Could you check a few things on this model? Use its own coordinates, in mm. Round coordinates to 2 decimals unless told otherwise and drop trailing zeros. Answer in a Markdown table with one row per item.
from build123d import *

# Parameters (mm, degrees)
SKETCH_1_R      = 2.103037388
EXTRUDE_1_DEPTH = 600


with BuildPart() as part:
    # 草图1 → 凸台-拉伸1 (new body)
    with BuildSketch(Plane.XY):
        with BuildLine():
            Line((-32.248557314, -0.229845073), (-32.248557314, -1.030984477))
            Line((-32.248557314, -1.030984477), (-33.250003689, -1.030984477))
            Line((-33.250003689, -1.030984477), (-33.250003689, -6.238394755))
            ThreePointArc((-33.250003689, -6.238394755), (-32.949991565, -6.938952391), (-32.24382973, -7.225524788))
            Line((-32.24382973, -7.225524788), (-27.078556151, -7.225524788))
            Line((-27.078556151, -7.225524788), (-27.078556151, -6.224078413))
            Line((-27.078556151, -6.224078413), (-26.277399051, -6.224078413))
            Line((-26.277399051, -6.224078413), (-26.277399051, -5.212715786))
            Line((-26.277399051, -5.212715786), (-29.27300496, -5.212715786))
            Line((-29.27300496, -5.212715786), (-29.27300496, -4.211495229))
            Line((-29.27300496, -4.211495229), (-26.279632969, -1.225390538))
            Line((-26.279632969, -1.225390538), (-20.24902045, -1.225390538))
            Line((-20.24902045, -1.225390538), (-17.255648459, -4.211495229))
            Line((-17.255648459, -4.211495229), (-17.255648459, -5.212715786))
            Line((-17.255648459, -5.212715786), (-20.251254368, -5.212715786))
            Line((-20.251254368, -5.212715786), (-20.251254368, -6.224078413))
            Line((-20.251254368, -6.224078413), (-19.450097268, -6.224078413))
            Line((-19.450097268, -6.224078413), (-19.450097268, -7.225524788))
            Line((-19.450097268, -7.225524788), (-7.064233131, -7.225524788))
            Line((-7.064233131, -7.225524788), (-7.064233131, -6.224078413))
            Line((-7.064233131, -6.224078413), (-6.263076031, -6.224078413))
            Line((-6.263076031, -6.224078413), (-6.263076031, -5.212715786))
            Line((-6.263076031, -5.212715786), (-9.25868194, -5.212715786))
            Line((-9.25868194, -5.212715786), (-9.25868194, -4.211495229))
            Line((-9.25868194, -4.211495229), (-6.265309949, -1.225390538))
            Line((-6.265309949, -1.225390538), (-0.234697429, -1.225390538))
            Line((-0.234697429, -1.225390538), (2.758674561, -4.211495229))
            Line((2.758674561, -4.211495229), (2.758674561, -5.212715786))
            Line((2.758674561, -5.212715786), (-0.236931348, -5.212715786))
            Line((-0.236931348, -5.212715786), (-0.236931348, -6.224078413))
            Line((-0.236931348, -6.224078413), (0.564225752, -6.224078413))
            Line((0.564225752, -6.224078413), (0.564225752, -7.225524788))
            Line((0.564225752, -7.225524788), (12.945482254, -7.225524788))
            Line((12.945482254, -7.225524788), (12.945482254, -6.219120287))
            Line((12.945482254, -6.219120287), (13.751246989, -6.219120287))
            Line((13.751246989, -6.219120287), (13.751246989, -5.212715786))
            Line((13.751246989, -5.212715786), (10.755641081, -5.212715786))
            Line((10.755641081, -5.212715786), (10.755641081, -4.211495229))
            Line((10.755641081, -4.211495229), (13.749013071, -1.225390538))
            Line((13.749013071, -1.225390538), (19.779625591, -1.225390538))
            Line((19.779625591, -1.225390538), (22.772997581, -4.211495229))
            Line((22.772997581, -4.211495229), (22.772997581, -5.212715786))
            Line((22.772997581, -5.212715786), (19.772784037, -5.212715786))
            Line((19.772784037, -5.212715786), (19.772784037, -6.219120287))
            Line((19.772784037, -6.219120287), (20.573941137, -6.219120287))
            Line((20.573941137, -6.219120287), (20.573941137, -7.225524788))
            Line((20.573941137, -7.225524788), (25.743822351, -7.225524788))
            ThreePointArc((25.743822351, -7.225524788), (26.449984187, -6.938952391), (26.749996311, -6.238394755))
            Line((26.749996311, -6.238394755), (26.749996311, -1.030984477))
            Line((26.749996311, -1.030984477), (25.748549936, -1.030984477))
            Line((25.748549936, -1.030984477), (25.748549936, -0.229827377))
            Line((25.748549936, -0.229827377), (24.761302481, -0.229827377))
            Line((24.761302481, -0.229827377), (24.761302481, -3.234203038))
            Line((24.761302481, -3.234203038), (23.759856106, -3.234203038))
            Line((23.759856106, -3.234203038), (20.770104831, -0.237175589))
            Line((20.770104831, -0.237175589), (20.770104831, 5.786126014))
            Line((20.770104831, 5.786126014), (23.759856106, 8.783153462))
            Line((23.759856106, 8.783153462), (24.761302481, 8.783153462))
            Line((24.761302481, 8.783153462), (24.761302481, 5.778777801))
            Line((24.761302481, 5.778777801), (25.748549936, 5.778777801))
            Line((25.748549936, 5.778777801), (25.748549936, 6.579934901))
            Line((25.748549936, 6.579934901), (26.749996311, 6.579934901))
            Line((26.749996311, 6.579934901), (26.749996311, 11.768212512))
            ThreePointArc((26.749996311, 11.768212512), (26.456722319, 12.481138347), (25.743822351, 12.774475212))
            Line((25.743822351, 12.774475212), (20.573941137, 12.774475212))
            Line((20.573941137, 12.774475212), (20.573941137, 11.768070711))
            Line((20.573941137, 11.768070711), (19.772784037, 11.768070711))
            Line((19.772784037, 11.768070711), (19.772784037, 10.761666211))
            Line((19.772784037, 10.761666211), (22.772997581, 10.761666211))
            Line((22.772997581, 10.761666211), (22.772997581, 9.760445653))
            Line((22.772997581, 9.760445653), (19.779625591, 6.774340962))
            Line((19.779625591, 6.774340962), (13.749013071, 6.774340962))
            Line((13.749013071, 6.774340962), (10.755641081, 9.760445653))
            Line((10.755641081, 9.760445653), (10.755641081, 10.761666211))
            Line((10.755641081, 10.761666211), (13.746639354, 10.761666211))
            Line((13.746639354, 10.761666211), (13.746639354, 11.768070711))
            Line((13.746639354, 11.768070711), (12.945482254, 11.768070711))
            Line((12.945482254, 11.768070711), (12.945482254, 12.774475212))
            Line((12.945482254, 12.774475212), (0.564225752, 12.774475212))
            Line((0.564225752, 12.774475212), (0.564225752, 11.773028837))
            Line((0.564225752, 11.773028837), (-0.236931348, 11.773028837))
            Line((-0.236931348, 11.773028837), (-0.236931348, 10.761666211))
            Line((-0.236931348, 10.761666211), (2.758674561, 10.761666211))
            Line((2.758674561, 10.761666211), (2.758674561, 9.760445653))
            Line((2.758674561, 9.760445653), (-0.234697429, 6.774340962))
            Line((-0.234697429, 6.774340962), (-6.265309949, 6.774340962))
            Line((-6.265309949, 6.774340962), (-9.25868194, 9.760445653))
            Line((-9.25868194, 9.760445653), (-9.25868194, 10.761666211))
            Line((-9.25868194, 10.761666211), (-6.263076031, 10.761666211))
            Line((-6.263076031, 10.761666211), (-6.263076031, 11.773028837))
            Line((-6.263076031, 11.773028837), (-7.064233131, 11.773028837))
            Line((-7.064233131, 11.773028837), (-7.064233131, 12.774475212))
            Line((-7.064233131, 12.774475212), (-19.450097268, 12.774475212))
            Line((-19.450097268, 12.774475212), (-19.450097268, 11.773028837))
            Line((-19.450097268, 11.773028837), (-20.251254368, 11.773028837))
            Line((-20.251254368, 11.773028837), (-20.251254368, 10.761666211))
            Line((-20.251254368, 10.761666211), (-17.255648459, 10.761666211))
            Line((-17.255648459, 10.761666211), (-17.255648459, 9.760445653))
            Line((-17.255648459, 9.760445653), (-20.24902045, 6.774340962))
            Line((-20.24902045, 6.774340962), (-26.279632969, 6.774340962))
            Line((-26.279632969, 6.774340962), (-29.27300496, 9.760445653))
            Line((-29.27300496, 9.760445653), (-29.27300496, 10.761666211))
            Line((-29.27300496, 10.761666211), (-26.277399051, 10.761666211))
            Line((-26.277399051, 10.761666211), (-26.277399051, 11.773028837))
            Line((-26.277399051, 11.773028837), (-27.078556151, 11.773028837))
            Line((-27.078556151, 11.773028837), (-27.078556151, 12.774475212))
            Line((-27.078556151, 12.774475212), (-32.24382973, 12.774475212))
            ThreePointArc((-32.24382973, 12.774475212), (-32.956729698, 12.481138347), (-33.250003689, 11.768212512))
            Line((-33.250003689, 11.768212512), (-33.250003689, 6.560802234))
            Line((-33.250003689, 6.560802234), (-32.248557314, 6.560802234))
            Line((-32.248557314, 6.560802234), (-32.248557314, 5.759645134))
            Line((-32.248557314, 5.759645134), (-31.261309859, 5.759645134))
            Line((-31.261309859, 5.759645134), (-31.261309859, 8.764020795))
            Line((-31.261309859, 8.764020795), (-30.259863484, 8.764020795))
            Line((-30.259863484, 8.764020795), (-27.27011221, 5.766993347))
            Line((-27.27011221, 5.766993347), (-27.27011221, -0.237175589))
            Line((-27.27011221, -0.237175589), (-30.259863484, -3.234203038))
            Line((-30.259863484, -3.234203038), (-31.261309859, -3.234203038))
            Line((-31.261309859, -3.234203038), (-31.261309859, -0.229845073))
            Line((-31.261309859, -0.229845073), (-32.248557314, -0.229845073))
        make_face()
        with Locations((-3.250003689, 2.774475212)):
            Circle(SKETCH_1_R, mode=Mode.SUBTRACT)
        with Locations((-23.250003689, 2.774475212)):
            Circle(SKETCH_1_R, mode=Mode.SUBTRACT)
        with Locations((16.749996311, 2.774475212)):
            Circle(SKETCH_1_R, mode=Mode.SUBTRACT)
        Polygon((-19.258541209, 5.786126014), (-19.258541209, -0.237175589), (-15.26734356, -4.238086639), (-15.26734356, -5.22228212), (-11.246986839, -5.22228212), (-11.246986839, -4.238086639), (-7.25578919, -0.237175589), (-7.25578919, 2.774475212), (-7.25578919, 5.786126014), (-11.246986839, 9.787037063), (-11.246986839, 10.771232544), (-15.26734356, 10.771232544), (-15.26734356, 9.787037063), align=None, mode=Mode.SUBTRACT)
        Polygon((4.74697946, -5.22228212), (8.767336181, -5.22228212), (8.767336181, -4.238086639), (12.758533831, -0.237175589), (12.758533831, 2.774475212), (12.758533831, 5.786126014), (8.767336181, 9.787037063), (8.767336181, 10.771232544), (4.74697946, 10.771232544), (4.74697946, 9.787037063), (0.755781811, 5.786126014), (0.755781811, 2.774475212), (0.755781811, -0.237175589), (4.74697946, -4.238086639), align=None, mode=Mode.SUBTRACT)
    extrude(amount=EXTRUDE_1_DEPTH)


solid = part.part
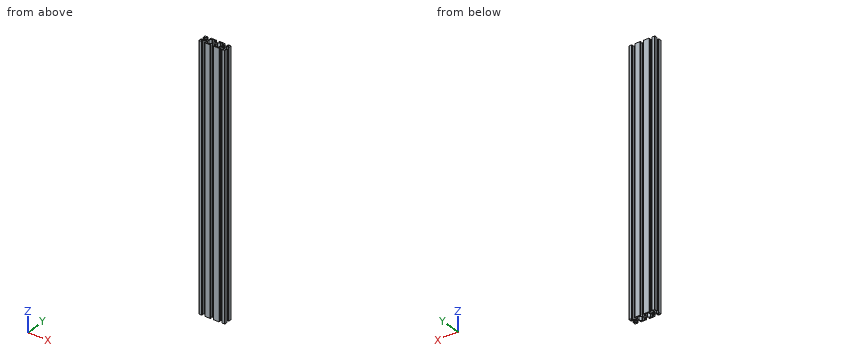
1) Imagine slicing it at A-A, the plane z = 432. Count the separate pieces of the cut face and the enclosed holes in it, plus the area to 3 significant figures.
Findings:
| item | result |
|---|---|
| separate pieces | 1 |
| enclosed holes | 5 |
| area | 448 mm^2 |
2) For pin 1 (5 mm diameter, centred on x = -22.5, z = 428.5, fed in from +Y); pin 2 (6 mm diameter, centred on x = 16.5, z = 338.5, fed in from -Y); pin 3 (10 mm diameter, centred on y = 4.5, z = 64.5, fed in from +X); pin 4 (4 mm diameter, centred on x = -3.25, y = 2.77, fed in from +Z), each with a flat end and sliding along its axis, tell me the tip position at first contact or that it passes through.
Findings:
| item | result |
|---|---|
| pin 1 | stops at y = 11.77 |
| pin 2 | stops at y = -6.22 |
| pin 3 | stops at x = 26.75 |
| pin 4 | passes through |
3) Please list where these lines run through material, in increasing order: line 1 (X direction, y = 3, z = 564); line 2 (X direction, y = 12, z = 307); line 3 (X direction, y = -4.25, z = 514.5).
Findings:
| item | result |
|---|---|
| line 1 | x = -27.27 to -25.34, -21.16 to -19.26, -7.26 to -5.34, -1.16 to 0.76, 12.76 to 14.66, 18.84 to 20.77 |
| line 2 | x = -33.22 to -27.08, -19.45 to -7.06, 0.56 to 12.95, 20.57 to 26.72 |
| line 3 | x = -33.25 to -29.27, -17.26 to -15.27, -11.25 to -9.26, 2.76 to 4.75, 8.77 to 10.76, 22.77 to 26.75 |
